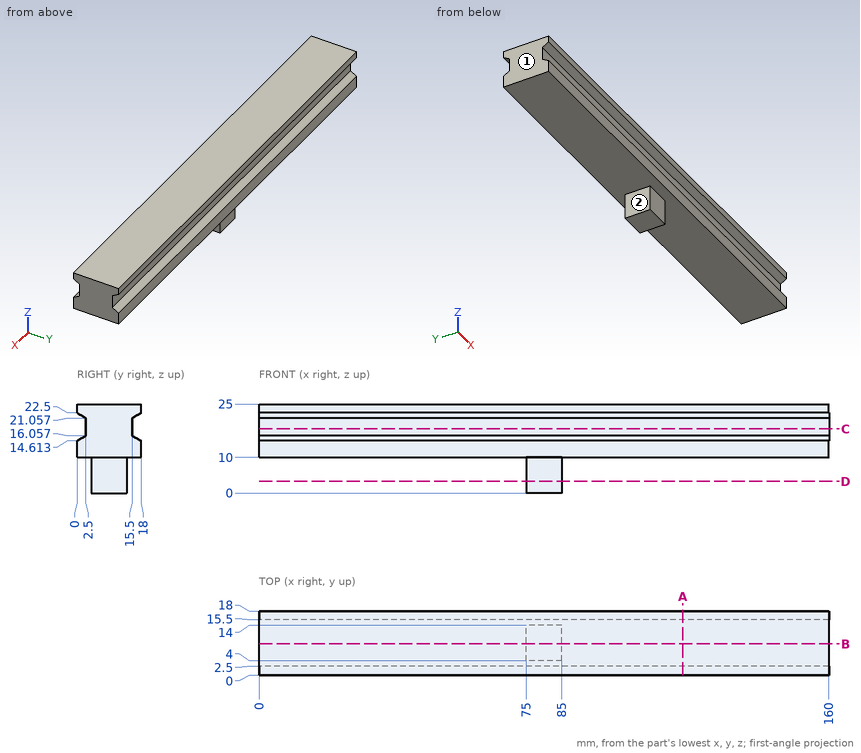
Design review of the part shown in the three views and the two pictorial views. Dimensions are in mm from the part's minimum x, y and z. A direction names the side the tool comes from. Round coordinates to 2 decimals unless told otherwise and drop trailing zeros. Loops run counter-clockwise (first coordinate to the right, second up) from the corner with the lowest first, then second, coordinate; pieces in that order, holes last. Notation, with made-up numbers: (-20, 15.5) -> (-1, 15.5) arc R19 ccw to (-1, 21.5) -> close; hole circle Ø11 at (-16.75, 47.5). An arc over 180 degrees is marked (long way). Use one line per item in the form item = value. Start each with the question number.
Q1. Wall thickness on line 1 along Z through (x, y) = (30.5, 12.25); line 2 along Z through (x, y) = (23, 15.75); line 3 along Y through (x, z) = (18, 20.25): over which ranges is each line inside the solid? List them lowest first. Write a range as [from, to].
Q2. Machinability: for the marked faces 1 and 2, which of the approach directions +Z, -Z, +X, -X, +Y, -Y give a long, thin tool a straight path to every point of the face, cutting with its end or side? Answer none if there is none.
Q3. For pin 1 Ø8 at (y, z) = (7, 4) entering from -X; pin 2 Ø5 at (x, z) = (79.5, 6.5) entering from -Y; pin 3 Ø8 at (y, z) = (7, 4) entering from +X, all flat-tipped, find the tip position at first contact; note any pin that passes through.
Q4. We need section B-B on y = 8.75. Give the boundary of the cut face in (x, z).
Q5. We need section D-D on z = 3.25. Give the boundary of the cut face in (x, y).
Q6. We need section A-A on x = 119. Give the boundary of the cut face in (y, z).
Q7. We need section C-C on z = 18. Give the boundary of the cut face in (x, y), then the cut area to 3 significant figures.
Calculated:
q1.line_1 = [10, 25]
q1.line_2 = [10, 15.91], [21.2, 25]
q1.line_3 = [2.5, 15.5]
q2.face_1 = +Z, -Z, -X, +Y, -Y
q2.face_2 = -Z, -X, +Y, -Y
q3.pin_1 = 75
q3.pin_2 = 4
q3.pin_3 = 85
q4.outline = (0, 10) -> (75, 10) -> (75, 0) -> (85, 0) -> (85, 10) -> (160, 10) -> (160, 25) -> (0, 25) -> close
q5.outline = (75, 4) -> (85, 4) -> (85, 14) -> (75, 14) -> close
q6.outline = (0, 10) -> (18, 10) -> (18, 14.61) -> (15.5, 16.06) -> (15.5, 21.06) -> (18, 22.5) -> (18, 25) -> (0, 25) -> (0, 22.5) -> (2.5, 21.06) -> (2.5, 16.06) -> (0, 14.61) -> close
q7.outline = (0, 2.5) -> (160, 2.5) -> (160, 15.5) -> (0, 15.5) -> close
q7.area = 2,080 mm²
